Input: part model. Units: mm. Frame: model coordinates. Face numbers are marked on the shaded views. A direction names the side the tool comes from. Round coordinates to 2 decimals unless told otherwise and drop trailing zeros. Loops run counter-clockwise (first coordinate to the right, second up) from the corner with the lowest first, then second, coordinate; pieces in that order, holes last.
(1) Line query: line 1 (Y direction, x = 41.5, z = -47.5); line 2 (X direction, y = 78, z = 23); line 3 (X direction, y = 68, z = -7.5). Output: solid intervals per line, ascending.
(2) Cut plane C-C, the plane y = 43.5. Output: boundary loops of the cut face in (x, z).
(3) First-contact query: pin 1 Ø2 at (y, z) = (84, -23) entering from +X (3 decimals); pin 2 Ø6 at (y, z) = (68.5, 30) entering from -X; pin 3 Ø12 at (x, z) = (-17.5, 32) entering from -Y; pin 4 Ø1.5 at (y, z) = (48.5, 7.5) entering from +X. Flat tips, straight axial feed; report the tip coordinate or a pass-through.
(4) Cut plane D-D, the plane x = 0. Output: boundary loops of the cut face in (y, z), and give its area (3 significant figures).
(5) Cut plane B-B, the plane x = 64. Output: boundary loops of the cut face in (y, z), and give its area (3 significant figures).
(6) Access query for the marked faces 1 and 2. Directions: +Z, -Z, +X, -X, +Y, -Y. A direction counts if a zero-diameter tool reaches every point of the face in a straight line with its end or side. Return the directions, or none.
(7) Cut plane A-A, the plane z = 0. Output: boundary loops of the cut face in (x, y).
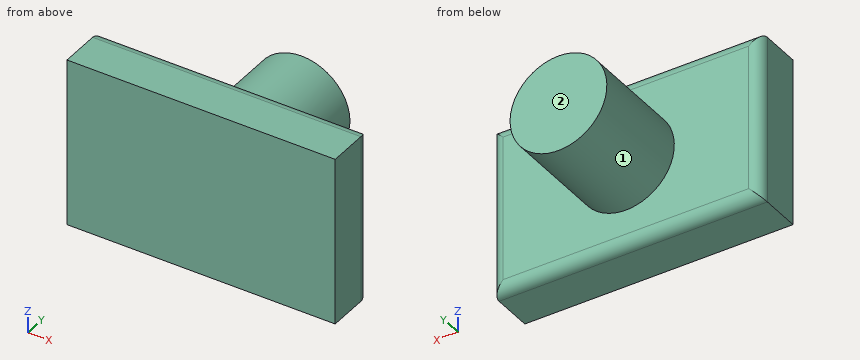
from build123d import *

# Parameters (mm, degrees)
SKETCH1_W           = 180.528529484
SKETCH1_H           = 113.389820172
BOSS_EXTRUDE1_DEPTH = 34.29
SKETCH3_R           = 32.56870091
BOSS_EXTRUDE2_DEPTH = 70.104
FILLET1_R           = 7.62


with BuildPart() as part:
    # Sketch1 → Boss-Extrude1 (new body)
    with BuildSketch(Plane(origin=(0, 0, 0), x_dir=(1, 0, 0), z_dir=(0, 1, 0))):
        Rectangle(SKETCH1_W, SKETCH1_H)
    extrude(amount=BOSS_EXTRUDE1_DEPTH)

    # Sketch3 → Boss-Extrude2 (add)
    with BuildSketch(Plane(origin=(0, 34.29, 0), x_dir=(1, 0, 0), z_dir=(0, 1, 0))):
        with Locations(Location((0, 0, 0), (0, 0, 270))):
            Circle(SKETCH3_R)
    extrude(amount=BOSS_EXTRUDE2_DEPTH)

    # Fillet1
    fillet1_edges = [part.edges().sort_by_distance(p)[0] for p in [
        (0, 34.29, -56.694910086),
        (-90.264264742, 34.29, 0),
        (0, 34.29, 56.694910086),
        (90.264264742, 34.29, 0),
    ]]
    fillet(fillet1_edges, radius=FILLET1_R)


solid = part.part
Reported:
1. line 1: y = 0 to 34.29
1. line 2: x = -23.06 to 23.06
1. line 3: x = -31.69 to 31.69
2. outline: circle Ø65.14 at (0, 0)
3. pin 1: stops at x = 24.015
3. pin 2: stops at x = -18.21
3. pin 3: stops at y = 0
3. pin 4: stops at x = 31.86
4. outline: (0, -56.69) - (26.67, -56.69) arc R7.62 ccw to (34.29, -49.07) - (34.29, -32.57) - (104.39, -32.57) - (104.39, 32.57) - (34.29, 32.57) - (34.29, 49.07) arc R7.62 ccw to (26.67, 56.69) - (0, 56.69) - close
4. area: 8,430 mm2
5. outline: (0, -56.69) - (26.67, -56.69) arc R7.62 ccw to (34.29, -49.07) - (34.29, 49.07) arc R7.62 ccw to (26.67, 56.69) - (0, 56.69) - close
5. area: 3,860 mm2
6. face 1: +Y
6. face 2: +Z, -Z, +X, -X, +Y
7. outline: (-90.26, 0) - (90.26, 0) - (90.26, 26.67) arc R7.62 ccw to (82.64, 34.29) - (32.57, 34.29) - (32.57, 104.39) - (-32.57, 104.39) - (-32.57, 34.29) - (-82.64, 34.29) arc R7.62 ccw to (-90.26, 26.67) - close
